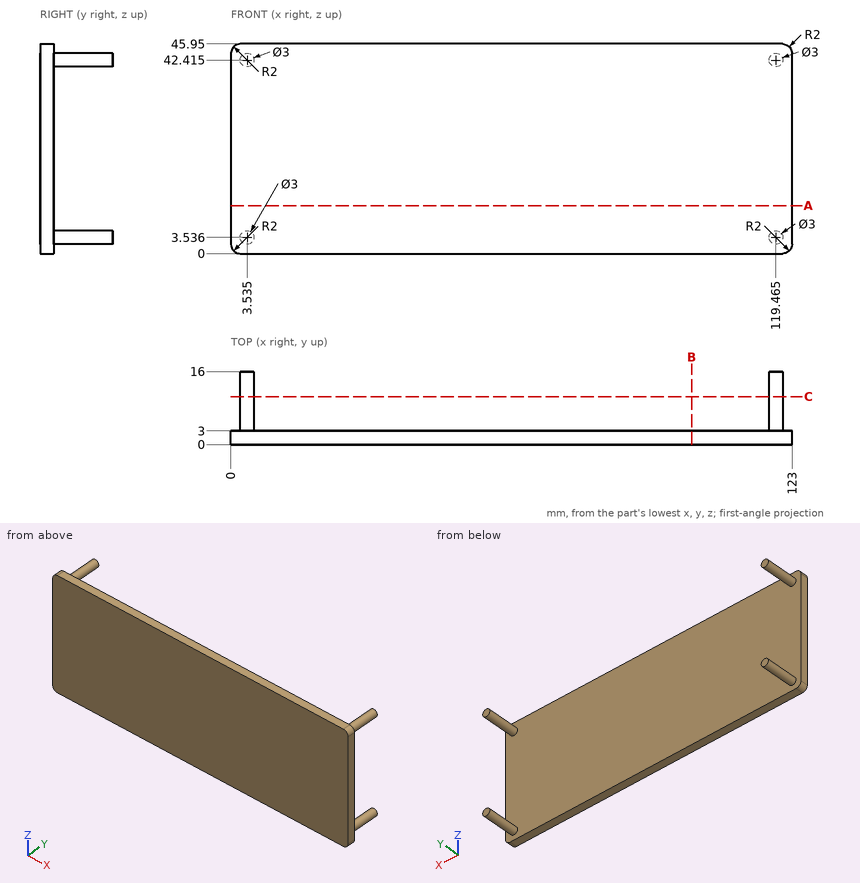
Part print with two shaded views. Sizes in mm from the minimum x, y, z corner. Round coordinates to 2 decimals unless told otherwise and drop trailing zeros. Loops run counter-clockwise (first coordinate to the right, second up) from the corner with the lowest first, then second, coordinate; pieces in that order, holes last. Notation, with made-up numbers: (13, 75.25) - (24, 75.25) arc R8 cw to (24, 85.25) - close; hole circle Ø3 at (-28, -14.75). An arc over 180 degrees is marked (long way). Put each result on its own line as item: value.
1. Slice it at A-A on z = 10.5. List the corners of the cut face in (x, y).
Geometry check:
outline: (0, 0) - (123, 0) - (123, 3) - (0, 3) - close
2. Wall check: line 1 (Y direction, x = 7, z = 10.5). Give the ranges that are in metal, low to high.
Geometry check:
line 1: 0 to 3
3. Slice it at C-C on y = 10.5. List the corners of the cut face in (x, z) (1 decimal).
Geometry check:
outline: circle Ø3 at (3.5, 3.5); circle Ø3 at (3.5, 42.4); circle Ø3 at (119.5, 3.5); circle Ø3 at (119.5, 42.4)
4. Pin check, flat tips, straight feed: P1, Ø1, axis at y = 8.5, z = 38.5, coming from the -X side; P2, Ø1.5, axis at x = 47, z = 38, coming from the +Y side. Stop position of each tip, or through.
Geometry check:
P1: through
P2: y = 3
5. Slice it at B-B on x = 101. List the corners of the cut face in (y, z), and give its area (3 significant figures).
Geometry check:
outline: (0, 0) - (3, 0) - (3, 45.95) - (0, 45.95) - close
area: 138 mm²
